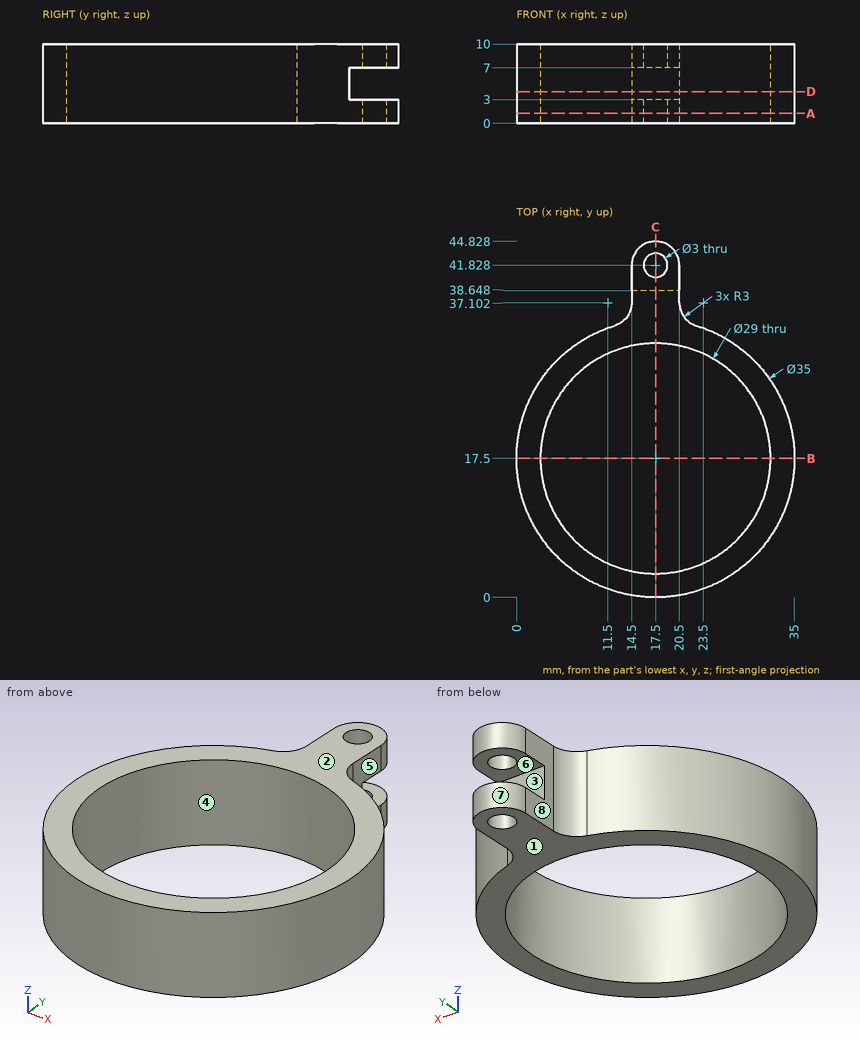
For this review, use the dimensioned drawing (mm, ordinates from the lowest corner) and the shaded views. A direction names the side the tool comes from. Give positions to 0.01 mm unless a question says otherwise; leave off trailing zeros. Write each loop counter-clockwise with the first axis right and the second up, starting at its lowest first coordinate (ties: lowest second). Pieces come first, ordered by that corner, then holes. Notation, with made-up numbers: M 62.25,81.5 L 103.25,81.5 A4 cw 103.25,88.5 Z; hole C 32.5,-33.5 d2. An arc over 180 degrees is marked long. Write item = value, one per line. Start each with the question number.
Q1. We need section A-A (z = 1.25). State the section outline as (x, y) points.
Q2. For line 1 (X direction, y = 18, z = 4.75); line 2 (Y direction, x = 17, z = 7.25) (1 decimal); line 3 (Y direction, x = 29, z = 2.25), list the stretches that pass through material, from the lowest coordinate up.
Q3. We need section C-C (x = 17.5). State the section outline as (y, z) points.
Q4. Machinability: for the marked faces 5, 6, 7 and 8, which of the approach directions +Z, -Z, +X, -X, +Y, -Y give a long, thin tool a straight path to every point of the face, cutting with its end or side? Answer none if there is none.
Q5. We need section D-D (z = 4). State the section outline as (x, y) points, plus the area to 3 significant figures.
Q6. Mouldability with a two-part tool opening along Z and no side actions: class the marked faces 1, 2, 3 and 4 as released by +Z, released by -Z, zero draft, split by the parting line, or undercut.
Q7. Clearance check with flat-ended pins moving along their axes: pin 1 (4 mm diameter, centred on y = 39.5, z = 4.5, fed in from -X); pin 2 (2.5 mm diameter, centred on x = 17.5, y = 41.83, fed in from -Z); pin 3 (4 mm diameter, centred on y = 39, z = 4, fed in from +X); pin 4 (4 mm diameter, centred on x = 29, z = 5.5, fed in from +Y). State where each tip first meets the part, or that it passes through.
Q8. We need section B-B (y = 17.5). State the section outline as (x, z) points, plus the area to 3 significant figures.
Result set:
q1.outline = M 12.38,34.23 A17.5 ccw long 22.62,34.23 A3 cw 20.5,37.1 L 20.5,41.83 A3 ccw 14.5,41.83 L 14.5,37.1 A3 cw Z; hole C 17.5,17.5 d29; hole C 17.5,41.83 d3
q2.line_1 = 0.01 to 3.01, 31.99 to 34.99
q2.line_2 = 0 to 3, 32 to 40.4, 43.2 to 44.8
q2.line_3 = 4.31 to 8.67, 26.33 to 30.69
q3.outline = M 0,0 L 3,0 L 3,10 L 0,10 Z; M 32,0 L 40.33,0 L 40.33,3 L 38.65,3 L 38.65,7 L 40.33,7 L 40.33,10 L 32,10 Z; M 43.33,0 L 44.83,0 L 44.83,3 L 43.33,3 Z; M 43.33,7 L 44.83,7 L 44.83,10 L 43.33,10 Z
q4.face_5 = +Z, -Z, +X, +Y
q4.face_6 = +X, -X, +Y
q4.face_7 = +Z, -Z, +Y
q4.face_8 = +Z, -Z, -X, +Y
q5.outline = M 12.38,34.23 A17.5 ccw long 22.62,34.23 A3 cw 20.5,37.1 L 20.5,38.65 L 14.5,38.65 L 14.5,37.1 A3 cw Z; hole C 17.5,17.5 d29
q5.area = 326 mm2
q6.face_1 = released by -Z
q6.face_2 = released by +Z
q6.face_3 = undercut
q6.face_4 = zero draft
q7.pin_1 = 14.5
q7.pin_2 = through
q7.pin_3 = 20.5
q7.pin_4 = 32.2
q8.outline = M 0,0 L 3,0 L 3,10 L 0,10 Z; M 32,0 L 35,0 L 35,10 L 32,10 Z
q8.area = 60.0 mm2
